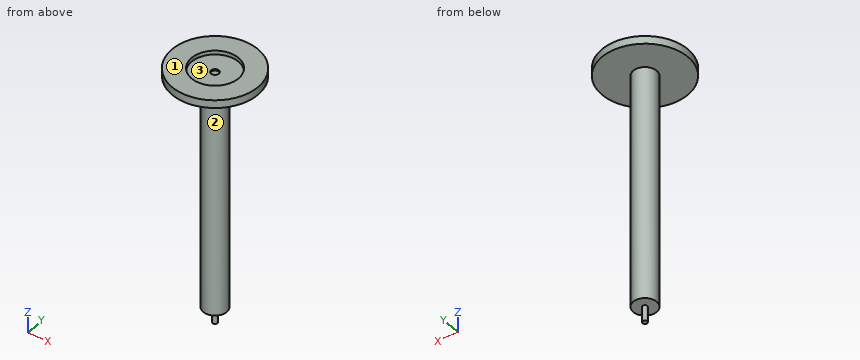
from build123d import *

# Parameters (mm, degrees)
SKETCH1_R           = 139.7
BOSS_EXTRUDE1_DEPTH = 25.4
SKETCH3_R           = 38.1
BOSS_EXTRUDE2_DEPTH = 762
SKETCH5_R           = 7.62
BOSS_EXTRUDE3_DEPTH = 50.8
SKETCH7_R           = 76.2
CUT_EXTRUDE1_DEPTH  = 12.7
SKETCH9_R           = 12.7
CUT_EXTRUDE3_DEPTH  = 5.08


with BuildPart() as part:
    # Sketch1 → Boss-Extrude1 (new body)
    with BuildSketch(Plane.XY):
        Circle(SKETCH1_R)
    extrude(amount=BOSS_EXTRUDE1_DEPTH)

    # Sketch3 → Boss-Extrude2 (add)
    with BuildSketch(Plane(origin=(0, 0, 0), x_dir=(-1, 0, 0), z_dir=(0, 0, -1))):
        with Locations(Location((0, 0, 0), (0, 0, 180))):
            Circle(SKETCH3_R)
    extrude(amount=BOSS_EXTRUDE2_DEPTH)

    # Sketch5 → Boss-Extrude3 (add)
    with BuildSketch(Plane(origin=(0, 0, -762), x_dir=(-1, 0, 0), z_dir=(0, 0, -1))):
        Circle(SKETCH5_R)
    extrude(amount=BOSS_EXTRUDE3_DEPTH)

    # Sketch7 → Cut-Extrude1 (cut)
    with BuildSketch(Plane.XY.offset(25.4)):
        Circle(SKETCH7_R)
    extrude(amount=-CUT_EXTRUDE1_DEPTH, mode=Mode.SUBTRACT)

    # Sketch9 → Cut-Extrude3 (cut)
    with BuildSketch(Plane.XY.offset(12.7)):
        Circle(SKETCH9_R)
    extrude(amount=-CUT_EXTRUDE3_DEPTH, mode=Mode.SUBTRACT)


solid = part.part
Could you check a few things on this model? Use its own coordinates, in mm. Face numbers are marked on the shaded views. Give positions to 0.01 mm unless a question says otherwise; leave off trailing zeros. Order: outer loops, then holes, each group sorted by start corner. A loop starts at its lowest first (then second) coordinate and runs counter-clockwise, first axis right, second up. Notation, with made-up numbers: (12, 3) - (32, 3) arc R11 ccw to (32, 14) - close; hole circle Ø3 at (71.5, 86). An arc over 180 degrees is marked (long way). One line per question, with ' | ' between items. Start each with the question number.
Item 1: I want a section at C-C on z = -236. Write out the boundary of the cut face in (x, y), then the cut area to 3 significant figures.
Item 2: I'm going to push flat-ended pins straight in: pin 1 Ø12 at (x, z) = (7, -253) entering from +Y; pin 2 Ø10 at (x, y) = (60.5, 92.5) entering from -Z; pin 3 Ø7.5 at (x, y) = (4.5, 6) entering from +Z. Where does each tip first touch, or does it pass through?
Item 3: Thinking about a two-plate mould opening in X: for the marked faces 1, 2 and 3, which applies, pulls with the +X half, pulls with the -X half, needs draft (parallel to the pull), parting line crosses it, or undercut?
Item 4: I want a section at A-A on x = 0. Write out the boundary of the cut face in (y, z).
Item 5: I want a section at D-D on y = 59. Write out the boundary of the cut face in (x, z), then the cut area to 3 significant figures.
Item 6: I need wall thicknesses on probe 1 along Y at (x, z) = (0, 17); probe 2 along Y at (x, z) = (0, 10); probe 3 along Z at (x, y) = (52, -52). Which ranges of each line are inside material? Lowest first, please. Write a range as [from, to].
Verdict:
1) outline: circle Ø76.2 at (0, 0) | area: 4,560 mm^2
2) pin 1: y = 38.09 | pin 2: z = 0 | pin 3: z = 7.62
3) face 1: needs draft | face 2: parting line crosses it | face 3: undercut
4) outline: (-139.7, 0) - (-38.1, 0) - (-38.1, -762) - (-7.62, -762) - (-7.62, -812.8) - (7.62, -812.8) - (7.62, -762) - (38.1, -762) - (38.1, 0) - (139.7, 0) - (139.7, 25.4) - (76.2, 25.4) - (76.2, 12.7) - (12.7, 12.7) - (12.7, 7.62) - (-12.7, 7.62) - (-12.7, 12.7) - (-76.2, 12.7) - (-76.2, 25.4) - (-139.7, 25.4) - close
5) outline: (-126.63, 0) - (126.63, 0) - (126.63, 25.4) - (48.22, 25.4) - (48.22, 12.7) - (-48.22, 12.7) - (-48.22, 25.4) - (-126.63, 25.4) - close | area: 5,210 mm^2
6) probe 1: [-139.7, -76.2], [76.2, 139.7] | probe 2: [-139.7, -12.7], [12.7, 139.7] | probe 3: [0, 12.7]
